For this review, take the finished solid that the model builds, in its own axes (mm). A direction names the side the tool comes from. Coordinates: 2 decimals unless noted, no trailing zeros. Order: outer loops, then holes, each group sorted by start corner. A loop starts at its lowest first (then second) coordinate and runs counter-clockwise, first axis right, second up. Notation, with made-up numbers: (36, 80.5) - (56, 80.5) arc R15 ccw to (56, 101.5) - close; hole circle Ø6 at (0, 45). An arc over 180 degrees is marked (long way). One line per item, written item: value. Start each with the question number.
(1) For faces 1 (the flat face through (-19, -12, -26.5)), 2 (the flat face through (-9, 24, 3)), 3 (the flat face through (0, -19, 53)), list the 3-axis set-ups (+Z, -Z, +X, -X, +Y, -Y) from which the entire face can be reached by the end or side of a thin tool; tool diameter is ignored.
(2) Mouldability with a two-part tool opening along X and no side actions: class faces 4 (the cylindrical face through (13.38, -25.73, 27.65)), 5 (the cylindrical face through (-16.812, -5.294, 0.779)), 6 (the flat face through (-15.2, 9.3, -50)) as released by +X, released by -X, zero draft, split by the parting line, or undercut.
(3) Consider section A-A on y = 0. Write out the cut boundary in (x, z).
(4) Clearance check with flat-ended pins moving along their axes: pin 1 (12 mm diameter, centred on x = -1.5, z = 1.5, fed in from +Y); pin 2 (8 mm diameter, centred on y = 18, z = 33.5, fed in from -X); pin 3 (6 mm diameter, centred on y = 7.5, z = 13, fed in from +X). State where each tip first meets the part, or that it passes through.
(5) Consider section D-D on z = -25. Write out the cut boundary in (x, y).
(6) To check wall thickness, follow line 1 along Y through (x, z) = (0, 8); line 2 along X through (y, z) = (-4, -15.5); line 3 along X through (y, z) = (0, -6.5). State the ranges of each line that lie inside material, in increasing order.
(7) Consider section C-C on z = 21. Write out the cut boundary in (x, y), then the cut area to 3 significant figures.
```python
from build123d import *

# Parameters (mm, degrees)
SKETCH1_R           = 20.625566824
BOSS_EXTRUDE1_DEPTH = 53
BOSS_EXTRUDE1_DRAFT = 5
SKETCH2_R           = 17.625566824
CUT_EXTRUDE1_DEPTH  = 64.917011631
SKETCH_4_R          = 29
SKETCH_4_R_2        = 17.625566824
EXTRUDE_1_DEPTH     = 50


with BuildPart() as part:
    # Sketch1 → Boss-Extrude1 (with draft: the straight prism first)
    with BuildSketch(Plane(origin=(0, 0, -50), x_dir=(-1, 0, 0), z_dir=(0, 0, -1))):
        Circle(SKETCH1_R)
    extrude(amount=-BOSS_EXTRUDE1_DEPTH)
    # Boss-Extrude1: the draft: its side faces are tilted about the plane it starts from
    boss_extrude1_sides = [part.faces().sort_by_distance(p)[0] for p in [
        (20.625566824, 0, -23.5),
    ]]
    draft(boss_extrude1_sides, Plane(origin=(0, 0, -50), x_dir=(-1, 0, 0), z_dir=(0, 0, -1)), BOSS_EXTRUDE1_DRAFT)

    # Sketch2 → Cut-Extrude1 (cut, through all)
    with BuildSketch(Plane(origin=(0, 0, -50), x_dir=(-1, 0, 0), z_dir=(0, 0, -1))):
        Circle(SKETCH2_R)
    extrude(amount=-CUT_EXTRUDE1_DEPTH, mode=Mode.SUBTRACT)

    # Эскиз1 → Вырез-Повернуть1 (revolve, cut)
    with BuildSketch(Plane(origin=(0, 0, 0), x_dir=(0, 0, -1), z_dir=(1, 0, 0)), mode=Mode.PRIVATE) as cut_revolve_1_sk:
        with BuildLine():
            Line((26.5, 22), (26.5, 23.5))
            Line((26.5, 23.5), (23.5, 23.5))
            Line((23.5, 23.5), (23.5, 22))
            ThreePointArc((23.5, 22), (25, 20.5), (26.5, 22))
        make_face()
    revolve(cut_revolve_1_sk.sketch.rotate(Axis((0, 0, -8.98762519), (0, 0, 1)), 90), axis=Axis((0, 0, -8.98762519), (0, 0, 1)), mode=Mode.SUBTRACT)

    # Эскиз4 → Бобышка-Вытянуть1 (add)
    with BuildSketch(Plane.XY.offset(3)):
        Circle(SKETCH_4_R)
        with Locations(Location((0, 0, 0), (0, 0, 180))):
            Circle(SKETCH_4_R_2, mode=Mode.SUBTRACT)
    extrude(amount=EXTRUDE_1_DEPTH)


solid = part.part
```
Geometry check:
1. face 1: none
1. face 2: -Z
1. face 3: +Z, +X, -X, +Y, -Y
2. face 4: split by the parting line
2. face 5: undercut
2. face 6: zero draft
3. outline: (-29, 3) - (-25.26, 3) - (-22.94, -23.5) - (-22, -23.5) arc R1.5 cw to (-22, -26.5) - (-22.68, -26.5) - (-20.63, -50) - (-17.63, -50) - (-17.63, 53) - (-29, 53) - close; (17.63, -50) - (20.63, -50) - (22.68, -26.5) - (22, -26.5) arc R1.5 cw to (22, -23.5) - (22.94, -23.5) - (25.26, 3) - (29, 3) - (29, 53) - (17.63, 53) - close
4. pin 1: stops at y = 29
4. pin 2: stops at x = -25.4
4. pin 3: stops at x = 28.65
5. outline: circle Ø41 at (0, 0); hole circle Ø35.25 at (0, 0)
6. line 1: y = -29 to -17.63, 17.63 to 29
6. line 2: x = -23.3 to -17.17, 17.17 to 23.3
6. line 3: x = -24.43 to -17.63, 17.63 to 24.43
7. outline: circle Ø58 at (0, 0); hole circle Ø35.25 at (0, 0)
7. area: 1,670 mm^2
